Part model, mm, in its own coordinate system. A direction names the side the tool comes from. Coordinates: 2 decimals unless noted, no trailing zeros. Order: outer loops, then holes, each group sorted by start corner. A loop starts at its lowest first (then second) coordinate and runs counter-clockwise, first axis right, second up.
1) Wall check: L1, parallel to Y at x = 0, z = 184. Give the ranges that are in metal, low to high.
2) Cut at B-B (z = 53.5). List the corners of the cut face in (x, y).
3) Mould opens along Y. For faces 1 (the flat face through (0, 4, 203)), 2 (the flat face through (0, -5, 197)), 3 (the flat face through (-5, 0, 197)) say: +Y half, -Y half, draft (parallel to the pull), parting line (faces both ways), or undercut.
4) Tool access for faces 4 (the flat face through (0, -4, 203)), 5 (the flat face through (-4.5, 0.1, 400)): list every direction of +Z, -Z, +X, -X, +Y, -Y with a clear straight run to the whole face (end or side of a thin tool).
5) Cut at A-A (x = -0.5). List the corners of the cut face in (y, z).
```python
from build123d import *

# Parameters (mm, degrees)
SKETCH2_W           = 10
SKETCH2_H           = 10
BOSS_EXTRUDE1_DEPTH = 400
SKETCH3_W           = 8
SKETCH3_H           = 8
CUT_EXTRUDE1_DEPTH  = 400


with BuildPart() as part:
    # Sketch2 → Boss-Extrude1 (new body)
    with BuildSketch(Plane.XY):
        Rectangle(SKETCH2_W, SKETCH2_H)
    extrude(amount=BOSS_EXTRUDE1_DEPTH)

    # Sketch3 → Cut-Extrude1 (cut)
    with BuildSketch(Plane.XY.offset(400)):
        Rectangle(SKETCH3_W, SKETCH3_H)
    extrude(amount=-CUT_EXTRUDE1_DEPTH, mode=Mode.SUBTRACT)


solid = part.part
```
Geometry check:
1. L1: y = -5 to -4, 4 to 5
2. outline: (-5, -5) - (5, -5) - (5, 5) - (-5, 5) - close; hole (-4, -4) - (4, -4) - (4, 4) - (-4, 4) - close
3. face 1: undercut
3. face 2: -Y half
3. face 3: draft
4. face 4: +Z, -Z
4. face 5: +Z, +X, -X, +Y, -Y
5. outline: (-5, 0) - (-4, 0) - (-4, 400) - (-5, 400) - close; (4, 0) - (5, 0) - (5, 400) - (4, 400) - close
